from build123d import *

# Parameters (mm, degrees)
SKETCH2_R           = 10
BOSS_EXTRUDE2_DEPTH = 15


with BuildPart() as part:
    # Sketch2 → Boss-Extrude2 (new body)
    with BuildSketch(Plane.XY):
        with BuildLine():
            Line((-230, 27), (230, 27))
            ThreePointArc((230, 27), (257, 0), (230, -27))
            Line((230, -27), (-230, -27))
            ThreePointArc((-230, -27), (-257, 0), (-230, 27))
        make_face()
        with Locations((-230, 0)):
            Circle(SKETCH2_R, mode=Mode.SUBTRACT)
        with Locations(Location((230, 0, 0), (0, 0, 180))):
            Circle(SKETCH2_R, mode=Mode.SUBTRACT)
    extrude(amount=-BOSS_EXTRUDE2_DEPTH)


solid = part.part
Work out the finished part from the listing and answer in its coordinate system (mm). Coordinates: 2 decimals unless noted, no trailing zeros. Write each loop counter-clockwise with the first axis right and the second up, starting at its lowest first coordinate (ties: lowest second). Pieces come first, ordered by that corner, then holes. Notation, with made-up numbers: (-37.75, -12) - (-17.75, -12) arc R35 cw to (-17.75, 24) - close; hole circle Ø5 at (53.5, -38). An arc over 180 degrees is marked (long way). One line per question, with ' | ' between items.
1) The mould has two halves that part along X. Classify faces 1 (the face through (256.993, 0.594, -7.395)), 2 (the face through (-256.993, -0.594, -7.395)), 3 (the face through (3, -27, -7)), 4 (the face through (220.763, 3.83, -7.395)): +X half, -X half, draft (parallel to the pull), parting line (faces both ways), or undercut.
Checks:
face 1: +X half | face 2: -X half | face 3: draft | face 4: undercut
2) Flat-ended cylindrical pins translate along their axes: P1, Ø8, axis at y = -12, z = -9.5, coming from the -X side; P2, Ø6, axis at y = -1.5, z = -1.5, coming from the -X side; P3, Ø6, axis at y = 13.5, z = -9, coming from the +X side. Find the tip coordinate at first contact, or state that the pin passes through.
Checks:
P1: x = -255.79 | P2: x = -257 | P3: x = 254.87
3) Find section B-B, the plane z = -5.25. Determine the outline of the cut face in (x, y).
Checks:
outline: (-230, -27) - (230, -27) arc R27 ccw to (230, 27) - (-230, 27) arc R27 ccw to start; hole circle Ø20 at (-230, 0); hole circle Ø20 at (230, 0)
4) Find section C-C, the plane y = -22.5. Determine the outline of the cut face in (x, z), and give its area (3 significant figures).
Checks:
outline: (-244.92, -15) - (244.92, -15) - (244.92, 0) - (-244.92, 0) - close | area: 7,350 mm2
5) Find section A-A, the plane y = 0. Determine the outline of the cut face in (x, z).
Checks:
outline: (-257, -15) - (-240, -15) - (-240, 0) - (-257, 0) - close; (-220, -15) - (220, -15) - (220, 0) - (-220, 0) - close; (240, -15) - (257, -15) - (257, 0) - (240, 0) - close
6) Consider probe 1 along Y at (x, z) = (230, -8.5); probe 2 along X at (y, z) = (-8, -2.25); probe 3 along X at (y, z) = (-3, -8.25). Determine where each line is inside the solid, lowest interval first. Write a range as [from, to].
Checks:
probe 1: [-27, -10], [10, 27] | probe 2: [-255.79, -236], [-224, 224], [236, 255.79] | probe 3: [-256.83, -239.54], [-220.46, 220.46], [239.54, 256.83]
